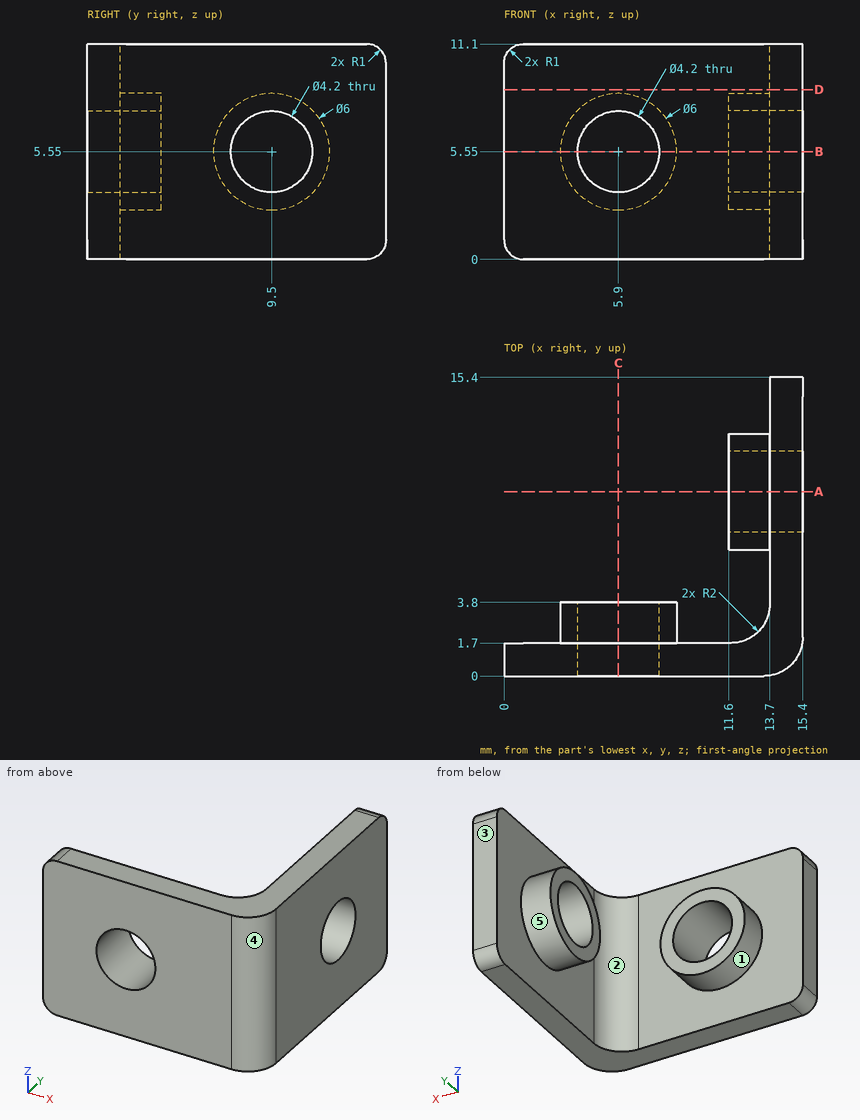
For this review, use the dimensioned drawing (mm, ordinates from the lowest corner) and the shaded views. A direction names the side the tool comes from. Coordinates: 2 decimals unless noted, no trailing zeros. Order: outer loops, then holes, each group sorted by start corner. A loop starts at its lowest first (then second) coordinate and runs counter-clockwise, first axis right, second up. Notation, with made-up numbers: (3.25, -25) -> (43.25, -25) arc R25 cw to (43.25, -12) -> close; hole circle Ø3 at (-21.5, -35.75). An arc over 180 degrees is marked (long way). One line per item, written item: value. Start each with the question number.
Q1. Mouldability with a two-part tool opening along Y and no side actions: class the marked faces 1, 2 and 3 as pulls with the +Y half, pulls with the -Y half, needs draft (parallel to the pull), parting line crosses it, or undercut.
Q2. Insertion check: pin 1 Ø5 at (y, z) = (10, 6.5) entering from -X; pin 2 Ø6.5 at (x, z) = (5, 5.5) entering from +Y; pin 3 Ø3.5 at (y, z) = (9.5, 5.55) entering from -X. Each pin has a flat end and moves straight along its axis. Give the tip position at first contact, or say it passes through.
Q3. Take a section at D-D, the plane z = 8.75. State the section outline as (x, y) points.
Q4. For probe 1 along X at (y, z) = (3.75, 5.5); probe 2 along Z at (x, y) = (5.9, 2.55); probe 3 along Y at (x, z) = (13.1, 5.55), list the stretches that pass through material, from the lowest coordinate up.
Q5. Take a section at B-B, the plane z = 5.55. State the section outline as (x, y) points, then the cut area to 4 significant figures.
Q6. Tool access review of the marked faces 4 and 5: name each direction out of +Z, -Z, +X, -X, +Y, -Y from which nothing blocks a thin tool from reaching the whole face with its end or side.
Q7. Take a section at C-C, the plane x = 5.9. State the section outline as (y, z) points.
Q8. Take a section at A-A, the plane y = 9.5. State the section outline as (x, z) points, then the cut area to 3 significant figures.
Values follow:
1. face 1: needs draft
1. face 2: undercut
1. face 3: pulls with the +Y half
2. pin 1: stops at x = 11.6
2. pin 2: stops at y = 3.8
2. pin 3: passes through
3. outline: (0, 0) -> (13.4, 0) arc R2 ccw to (15.4, 2) -> (15.4, 15.4) -> (13.7, 15.4) -> (13.7, 3.7) arc R2 cw to (11.7, 1.7) -> (0, 1.7) -> close
4. probe 1: x = 2.9 to 3.8, 8 to 8.9, 13.7 to 15.4
4. probe 2: z = 2.55 to 3.45, 7.65 to 8.55
4. probe 3: y = 0 to 2.27, 6.5 to 7.4, 11.6 to 12.5
5. outline: (0, 0) -> (3.8, 0) -> (3.8, 3.8) -> (2.9, 3.8) -> (2.9, 1.7) -> (0, 1.7) -> close; (8, 0) -> (13.4, 0) arc R2 ccw to (15.4, 2) -> (15.4, 7.4) -> (11.6, 7.4) -> (11.6, 6.5) -> (13.7, 6.5) -> (13.7, 3.7) arc R2 cw to (11.7, 1.7) -> (8.9, 1.7) -> (8.9, 3.8) -> (8, 3.8) -> close; (11.6, 11.6) -> (15.4, 11.6) -> (15.4, 15.4) -> (13.7, 15.4) -> (13.7, 12.5) -> (11.6, 12.5) -> close
5. area: 42.75 mm2
6. face 4: +Z, -Z, +X, -Y
6. face 5: -X
7. outline: (0, 0) -> (1.7, 0) -> (1.7, 2.55) -> (3.8, 2.55) -> (3.8, 3.45) -> (0, 3.45) -> close; (0, 7.65) -> (3.8, 7.65) -> (3.8, 8.55) -> (1.7, 8.55) -> (1.7, 11.1) -> (0, 11.1) -> close
8. outline: (11.6, 2.55) -> (13.7, 2.55) -> (13.7, 0) -> (15.4, 0) -> (15.4, 3.45) -> (11.6, 3.45) -> close; (11.6, 7.65) -> (15.4, 7.65) -> (15.4, 11.1) -> (13.7, 11.1) -> (13.7, 8.55) -> (11.6, 8.55) -> close
8. area: 15.5 mm2
